Here's how the part is built. I have some questions about the finished solid (model axes, mm). Face numbers are marked on the shaded views. Round coordinates to 2 decimals unless told otherwise and drop trailing zeros. Loops run counter-clockwise (first coordinate to the right, second up) from the corner with the lowest first, then second, coordinate; pieces in that order, holes last. Notation, with made-up numbers: M 12,56.25 L 28,56.25 A18 ccw 28,83.25 Z; hole C 7.5,-38 d4. An arc over 180 degrees is marked long. Answer as a JSON object with one key per item and string values.
from build123d import *

# Parameters (mm, degrees)
F0_R     = 25.4
F1_DEPTH = 6.35
F2_R     = 3.81
F4_R     = 19.2670598269
F5_DEPTH = 1.27
F6_R     = 0.8432395902
F7_DEPTH = 0.762
F8_R     = 1.5748
F8_R_2   = 0.8432395902
F9_DEPTH = 0.127
F10_R    = 0.12699


# Not quite as in the source:
# - a fillet or chamfer that OpenCascade refuses, or shapes differently, is made with other operations: its cross-section is extruded or revolved along the edge and cut away or added
# - a fillet or chamfer is up to 0.001 mm smaller than in the source, because OpenCascade refuses the exact size


with BuildPart() as f1:
    # F0 (on Top) → F1 (new body)
    with BuildSketch(Plane.XY):
        Circle(F0_R)
    extrude(amount=F1_DEPTH)

    # F2
    f2_edges = [f1.edges().sort_by_distance(p)[0] for p in [
        (-25.4, 0, 0),
    ]]
    fillet(f2_edges, radius=F2_R)

    # F3: fillet of radius 5.08 on 1 edges, made by hand

    # F3_s1 → F3_t2 (revolve, cut)
    with BuildSketch(Plane.XZ):
        with BuildLine():
            ThreePointArc((25.4, 3.81), (23.5405909488, 5.6694090512), (21.0005909488, 6.35))
            Line((21.0005909488, 6.35), (25.4, 6.35))
            Line((25.4, 6.35), (25.4, 3.81))
        make_face()
    revolve(axis=Axis((0, 0, 6.35), (0, 0, 1)), mode=Mode.SUBTRACT)

    # F4 (on face) → F5 (cut)
    with BuildSketch(Plane.XY.offset(6.35)):
        Circle(F4_R)
    extrude(amount=-F5_DEPTH, mode=Mode.SUBTRACT)

    # F6 (on face) → F7 (join)
    with BuildSketch(Plane.XY.offset(5.08)):
        Circle(F6_R)
    extrude(amount=F7_DEPTH)

    # F8 (on face) → F9 (join)
    with BuildSketch(Plane.XY.offset(5.842)):
        Circle(F8_R)
        Circle(F8_R_2, mode=Mode.SUBTRACT)
        Circle(F8_R_2)
    extrude(amount=F9_DEPTH)

    # F10 (radius 0.127 in the source; OpenCascade refuses exactly that, so slightly less here)
    f10_edges = [f1.edges().sort_by_distance(p)[0] for p in [
        (-1.5748, 0, 5.969),
    ]]
    fillet(f10_edges, radius=F10_R)


solid = f1.part
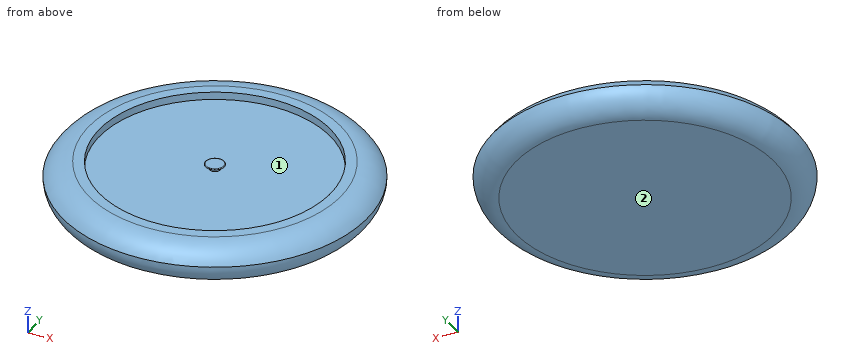
Item 1: I want a section at C-C on z = 1. List the corners of the cut face in (x, y) for me.
Solution:
{"outline": "C 0,0 d48.33"}
Item 2: If I drill on L1, parallel to Y at x = 0, z = 5.4; L2, parallel to Y at x = 0, z = 5.9; L3, parallel to Z at x = -13, y = -6, over which ranges is the centre line in solid material (lowest first)? Write a range as from..to.
Solution:
{"L1": "y = -23.96..-19.27, -0.84..0.84, 19.27..23.96", "L2": "y = -23.09..-19.27, -1.56..1.56, 19.27..23.09", "L3": "z = 0..5.08"}
Item 3: We'd pull the mould along Y, two halves only. Please class the marked faces 1 and 2: +Y half, -Y half, draft (parallel to the pull), parting line (faces both ways), or undercut.
Solution:
{"face 1": "undercut", "face 2": "draft"}
Item 4: For P1, Ø1.5, axis at x = 1, y = 0.5, coming from the +Z side; P2, Ø2, axis at y = 14.5, z = 4, coming from the -X side, each with a flat end and sliding along its axis, tell me the tip position at first contact or that it passes through.
Solution:
{"P1": "stops at z = 5.97", "P2": "stops at x = -21.5"}
